Check sheet for the modelled part. Datum: model origin and axes. Units: mm. Round coordinates to 2 decimals unless told otherwise and drop trailing zeros. Write each loop counter-clockwise with the first axis right and the second up, starting at its lowest first coordinate (ties: lowest second). Pieces come first, ordered by that corner, then holes. Notation, with made-up numbers: (27, -20) -> (73, -20) arc R25 cw to (73, 16) -> close; hole circle Ø1 at (-37.75, 11). An arc over 180 degrees is marked (long way). One line per item, written item: value.
from build123d import *

# Parameters (mm, degrees)
SKETCH1_W           = 720
SKETCH1_H           = 409
BOSS_EXTRUDE1_DEPTH = 3
CUT_EXTRUDE2_DEPTH  = 415.072759307
CUT_EXTRUDE3_DEPTH  = 415.072759307
SKETCH7_R           = 2.25
CUT_EXTRUDE4_DEPTH  = 415.072759307
SKETCH9_R           = 43
CUT_EXTRUDE6_DEPTH  = 415.072759308


with BuildPart() as part:
    # Sketch1 → Boss-Extrude1 (new, symmetric)
    with BuildSketch(Plane(origin=(0, 0, 0), x_dir=(1, 0, 0), z_dir=(0, 1, 0))):
        Rectangle(SKETCH1_W, SKETCH1_H)
    extrude(amount=BOSS_EXTRUDE1_DEPTH, both=True)

    # Sketch5 → Cut-Extrude2 (cut, through all)
    with BuildSketch(Plane(origin=(0, 3, 0), x_dir=(1, 0, 0), z_dir=(0, 1, 0))):
        with BuildLine():
            Line((154, 79.5), (171, 79.5))
            ThreePointArc((171, 79.5), (173.828427125, 78.328427125), (175, 75.5))
            Line((175, 75.5), (175, -66.5))
            ThreePointArc((175, -66.5), (173.828427125, -69.328427125), (171, -70.5))
            Line((171, -70.5), (154, -70.5))
            ThreePointArc((154, -70.5), (151.171572875, -69.328427125), (150, -66.5))
            Line((150, -66.5), (150, 75.5))
            ThreePointArc((150, 75.5), (151.171572875, 78.328427125), (154, 79.5))
        make_face()
    extrude(amount=-CUT_EXTRUDE2_DEPTH, mode=Mode.SUBTRACT)

    # Sketch6 → Cut-Extrude3 (cut, through all)
    with BuildSketch(Plane(origin=(0, 3, 0), x_dir=(1, 0, 0), z_dir=(0, 1, 0))):
        with BuildLine():
            Line((-360, 204.5), (-319, 204.5))
            Line((-319, 204.5), (-319, 174.5))
            ThreePointArc((-319, 174.5), (-320.171572875, 171.671572875), (-323, 170.5))
            Line((-323, 170.5), (-360, 170.5))
            Line((-360, 170.5), (-360, 204.5))
        make_face()
    extrude(amount=-CUT_EXTRUDE3_DEPTH, mode=Mode.SUBTRACT)

    # Sketch7 → Cut-Extrude4 (cut, through all)
    with BuildSketch(Plane(origin=(0, 3, 0), x_dir=(1, 0, 0), z_dir=(0, 1, 0))):
        with Locations(Location((-260, 189.5, 0), (0, 0, 270))):
            Circle(SKETCH7_R)
        with Locations(Location((25, 189.5, 0), (0, 0, 270))):
            Circle(SKETCH7_R)
        with Locations(Location((310, 189.5, 0), (0, 0, 270))):
            Circle(SKETCH7_R)
        with Locations(Location((310, -160.5, 0), (0, 0, 90))):
            Circle(SKETCH7_R)
        with Locations(Location((25, -160.5, 0), (0, 0, 90))):
            Circle(SKETCH7_R)
        with Locations(Location((-260, -160.5, 0), (0, 0, 90))):
            Circle(SKETCH7_R)
        with Locations(Location((-200, 152, 0), (0, 0, 270))):
            Circle(SKETCH7_R)
        with Locations(Location((-200, -123, 0), (0, 0, 270))):
            Circle(SKETCH7_R)
        with Locations(Location((-80, 152, 0), (0, 0, 270))):
            Circle(SKETCH7_R)
        with Locations(Location((-80, -123, 0), (0, 0, 270))):
            Circle(SKETCH7_R)
        with Locations(Location((40, 152, 0), (0, 0, 270))):
            Circle(SKETCH7_R)
        with Locations(Location((40, -123, 0), (0, 0, 270))):
            Circle(SKETCH7_R)
        with Locations(Location((182.5, 87, 0), (0, 0, 270))):
            Circle(SKETCH7_R)
        with Locations(Location((242.5, 87, 0), (0, 0, 270))):
            Circle(SKETCH7_R)
        with Locations(Location((242.5, -78, 0), (0, 0, 270))):
            Circle(SKETCH7_R)
        with Locations(Location((182.5, -78, 0), (0, 0, 270))):
            Circle(SKETCH7_R)
    extrude(amount=-CUT_EXTRUDE4_DEPTH, mode=Mode.SUBTRACT)

    # Cut-Extrude5 cone 1 section (through the dimple's axis) → Cut-Extrude5 (revolve, cut)
    with BuildSketch(Plane(origin=(-260, 3, -189.5), x_dir=(0, 0, 1), z_dir=(1, 0, 0))):
        Polygon((0, 0), (4.5, 0), (0, 4.5), align=None)
    revolve(axis=Axis((-260, 3, -189.5), (0, -1, 0)), mode=Mode.SUBTRACT)

    # Cut-Extrude5 cone 2 section (through the dimple's axis) → Cut-Extrude5 cone 2 (revolve, cut)
    with BuildSketch(Plane(origin=(-200, 3, -152), x_dir=(0, 0, 1), z_dir=(1, 0, 0))):
        Polygon((0, 0), (4.5, 0), (0, 4.5), align=None)
    revolve(axis=Axis((-200, 3, -152), (0, -1, 0)), mode=Mode.SUBTRACT)

    # Cut-Extrude5 cone 3 section (through the dimple's axis) → Cut-Extrude5 cone 3 (revolve, cut)
    with BuildSketch(Plane(origin=(-80, 3, -152), x_dir=(0, 0, 1), z_dir=(1, 0, 0))):
        Polygon((0, 0), (4.5, 0), (0, 4.5), align=None)
    revolve(axis=Axis((-80, 3, -152), (0, -1, 0)), mode=Mode.SUBTRACT)

    # Cut-Extrude5 cone 4 section (through the dimple's axis) → Cut-Extrude5 cone 4 (revolve, cut)
    with BuildSketch(Plane(origin=(25, 3, -189.5), x_dir=(0, 0, 1), z_dir=(1, 0, 0))):
        Polygon((0, 0), (4.5, 0), (0, 4.5), align=None)
    revolve(axis=Axis((25, 3, -189.5), (0, -1, 0)), mode=Mode.SUBTRACT)

    # Cut-Extrude5 cone 5 section (through the dimple's axis) → Cut-Extrude5 cone 5 (revolve, cut)
    with BuildSketch(Plane(origin=(40, 3, -152), x_dir=(0, 0, 1), z_dir=(1, 0, 0))):
        Polygon((0, 0), (4.5, 0), (0, 4.5), align=None)
    revolve(axis=Axis((40, 3, -152), (0, -1, 0)), mode=Mode.SUBTRACT)

    # Cut-Extrude5 cone 6 section (through the dimple's axis) → Cut-Extrude5 cone 6 (revolve, cut)
    with BuildSketch(Plane(origin=(310, 3, -189.5), x_dir=(0, 0, 1), z_dir=(1, 0, 0))):
        Polygon((0, 0), (4.5, 0), (0, 4.5), align=None)
    revolve(axis=Axis((310, 3, -189.5), (0, -1, 0)), mode=Mode.SUBTRACT)

    # Cut-Extrude5 cone 7 section (through the dimple's axis) → Cut-Extrude5 cone 7 (revolve, cut)
    with BuildSketch(Plane(origin=(-200, 3, 123), x_dir=(0, 0, 1), z_dir=(1, 0, 0))):
        Polygon((0, 0), (4.5, 0), (0, 4.5), align=None)
    revolve(axis=Axis((-200, 3, 123), (0, -1, 0)), mode=Mode.SUBTRACT)

    # Cut-Extrude5 cone 8 section (through the dimple's axis) → Cut-Extrude5 cone 8 (revolve, cut)
    with BuildSketch(Plane(origin=(-260, 3, 160.5), x_dir=(0, 0, 1), z_dir=(1, 0, 0))):
        Polygon((0, 0), (4.5, 0), (0, 4.5), align=None)
    revolve(axis=Axis((-260, 3, 160.5), (0, -1, 0)), mode=Mode.SUBTRACT)

    # Cut-Extrude5 cone 9 section (through the dimple's axis) → Cut-Extrude5 cone 9 (revolve, cut)
    with BuildSketch(Plane(origin=(-80, 3, 123), x_dir=(0, 0, 1), z_dir=(1, 0, 0))):
        Polygon((0, 0), (4.5, 0), (0, 4.5), align=None)
    revolve(axis=Axis((-80, 3, 123), (0, -1, 0)), mode=Mode.SUBTRACT)

    # Cut-Extrude5 cone 10 section (through the dimple's axis) → Cut-Extrude5 cone 10 (revolve, cut)
    with BuildSketch(Plane(origin=(25, 3, 160.5), x_dir=(0, 0, 1), z_dir=(1, 0, 0))):
        Polygon((0, 0), (4.5, 0), (0, 4.5), align=None)
    revolve(axis=Axis((25, 3, 160.5), (0, -1, 0)), mode=Mode.SUBTRACT)

    # Cut-Extrude5 cone 11 section (through the dimple's axis) → Cut-Extrude5 cone 11 (revolve, cut)
    with BuildSketch(Plane(origin=(40, 3, 123), x_dir=(0, 0, 1), z_dir=(1, 0, 0))):
        Polygon((0, 0), (4.5, 0), (0, 4.5), align=None)
    revolve(axis=Axis((40, 3, 123), (0, -1, 0)), mode=Mode.SUBTRACT)

    # Cut-Extrude5 cone 12 section (through the dimple's axis) → Cut-Extrude5 cone 12 (revolve, cut)
    with BuildSketch(Plane(origin=(310, 3, 160.5), x_dir=(0, 0, 1), z_dir=(1, 0, 0))):
        Polygon((0, 0), (4.5, 0), (0, 4.5), align=None)
    revolve(axis=Axis((310, 3, 160.5), (0, -1, 0)), mode=Mode.SUBTRACT)

    # Cut-Extrude5 cone 13 section (through the dimple's axis) → Cut-Extrude5 cone 13 (revolve, cut)
    with BuildSketch(Plane(origin=(182.5, 3, -87), x_dir=(0, 0, 1), z_dir=(1, 0, 0))):
        Polygon((0, 0), (4.5, 0), (0, 4.5), align=None)
    revolve(axis=Axis((182.5, 3, -87), (0, -1, 0)), mode=Mode.SUBTRACT)

    # Cut-Extrude5 cone 14 section (through the dimple's axis) → Cut-Extrude5 cone 14 (revolve, cut)
    with BuildSketch(Plane(origin=(242.5, 3, -87), x_dir=(0, 0, 1), z_dir=(1, 0, 0))):
        Polygon((0, 0), (4.5, 0), (0, 4.5), align=None)
    revolve(axis=Axis((242.5, 3, -87), (0, -1, 0)), mode=Mode.SUBTRACT)

    # Cut-Extrude5 cone 15 section (through the dimple's axis) → Cut-Extrude5 cone 15 (revolve, cut)
    with BuildSketch(Plane(origin=(182.5, 3, 78), x_dir=(0, 0, 1), z_dir=(1, 0, 0))):
        Polygon((0, 0), (4.5, 0), (0, 4.5), align=None)
    revolve(axis=Axis((182.5, 3, 78), (0, -1, 0)), mode=Mode.SUBTRACT)

    # Cut-Extrude5 cone 16 section (through the dimple's axis) → Cut-Extrude5 cone 16 (revolve, cut)
    with BuildSketch(Plane(origin=(242.5, 3, 78), x_dir=(0, 0, 1), z_dir=(1, 0, 0))):
        Polygon((0, 0), (4.5, 0), (0, 4.5), align=None)
    revolve(axis=Axis((242.5, 3, 78), (0, -1, 0)), mode=Mode.SUBTRACT)

    # Sketch9 → Cut-Extrude6 (cut, through all)
    with BuildSketch(Plane(origin=(0, 3, 0), x_dir=(1, 0, 0), z_dir=(0, 1, 0))):
        with Locations(Location((-20, 4.5, 0), (0, 0, 270))):
            Circle(SKETCH9_R)
        with Locations(Location((-140, 4.5, 0), (0, 0, 270))):
            Circle(SKETCH9_R)
    extrude(amount=-CUT_EXTRUDE6_DEPTH, mode=Mode.SUBTRACT)


solid = part.part
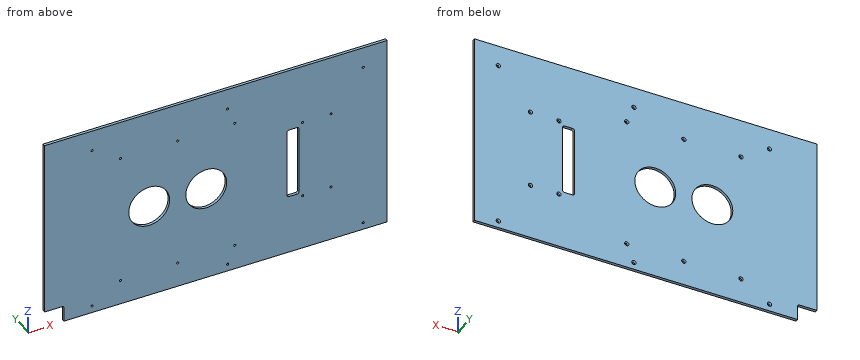
Item 1: Sectioned sample at C-C on y = -1.35. Count the separate pieces of the cut face and the enclosed holes in it, and give its area (3 significant figures).
Answer:
separate pieces: 1
enclosed holes: 19
area: 277,000 mm^2
Item 2: Depth check by flat-ended pin: P1, Ø6, axis at x = 25, z = -189.5, coming from the +Y side. Enter the tip coordinate at first touch or a pass-through.
Answer:
P1: stops at y = 1.5
Item 3: Thickness scan on line 1 (X direction, y = -1.35, z = -87); line 2 (Z direction, x = -260, y = -0.9); line 3 (X direction, y = -1.3, z = -189.5). Record the ranges inside material, lowest first.
Answer:
line 1: x = -360 to 180.25, 184.75 to 240.25, 244.75 to 360
line 2: z = -204.5 to -191.75, -187.25 to 158.25, 162.75 to 204.5
line 3: x = -319 to -262.25, -257.75 to 22.75, 27.25 to 307.75, 312.25 to 360
Item 4: Sectioned sample at B-B on x = -157.5. Enter the section's corners in (y, z), and give its area (3 significant figures).
Answer:
outline: (-3, -204.5) -> (3, -204.5) -> (3, -43.78) -> (-3, -43.78) -> close; (-3, 34.78) -> (3, 34.78) -> (3, 204.5) -> (-3, 204.5) -> close
area: 1,980 mm^2
Item 5: Sectioned sample at D-D on z = -1.5. Enter the section's corners in (x, y), and give its area (3 significant figures).
Answer:
outline: (-360, -3) -> (-182.9, -3) -> (-182.9, 3) -> (-360, 3) -> close; (-97.1, -3) -> (-62.9, -3) -> (-62.9, 3) -> (-97.1, 3) -> close; (22.9, -3) -> (150, -3) -> (150, 3) -> (22.9, 3) -> close; (175, -3) -> (360, -3) -> (360, 3) -> (175, 3) -> close
area: 3,140 mm^2
Item 6: Sectioned sample at A-A on z = -64.5. Enter the section's corners in (x, y).
Answer:
outline: (-360, -3) -> (150, -3) -> (150, 3) -> (-360, 3) -> close; (175, -3) -> (360, -3) -> (360, 3) -> (175, 3) -> close
